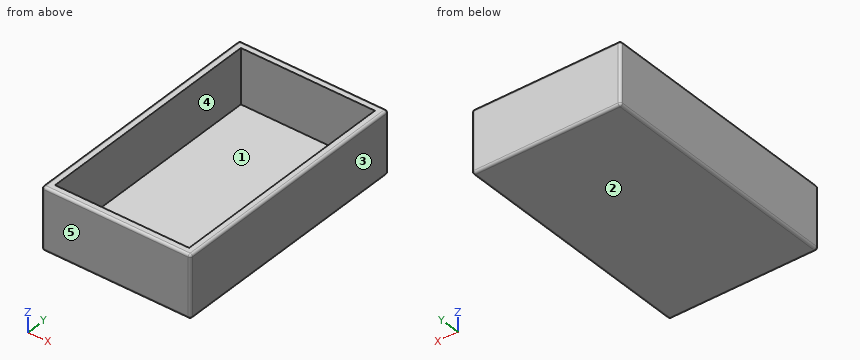
```python
from build123d import *

# Parameters (mm, degrees)
F0_W     = 60
F0_H     = 100
F1_DEPTH = 25
F2_T     = -3
F3_R     = 1


with BuildPart() as f1:
    # F0 (on Top) → F1 (new body)
    with BuildSketch(Plane.XY):
        with Locations((-16.971023, 0.550396)):
            Rectangle(F0_W, F0_H)
    extrude(amount=F1_DEPTH)

    # F2
    f2_openings = [f1.faces().sort_by_distance(p)[0] for p in [
        (-16.971023, 0.550396, 25),
    ]]
    offset(amount=F2_T, openings=f2_openings)

    # F3
    f3_edges = [f1.edges().sort_by_distance(p)[0] for p in [
        (13.028977, 0.550396, 25),
        (-16.971023, -49.449604, 25),
        (-46.971023, 0.550396, 25),
        (-16.971023, 50.550396, 25),
        (13.028977, 50.550396, 12.5),
        (13.028977, -49.449604, 12.5),
        (-46.971023, -49.449604, 12.5),
        (-16.971023, -49.449604, 0),
        (13.028977, 0.550396, 0),
        (-16.971023, 50.550396, 0),
        (-46.971023, 0.550396, 0),
        (-46.971023, 50.550396, 12.5),
    ]]
    fillet(f3_edges, radius=F3_R)


solid = f1.part
```
Could you check a few things on this model? Use its own coordinates, in mm. Face numbers are marked on the shaded views. A direction names the side the tool comes from. Round coordinates to 2 decimals unless told otherwise and drop trailing zeros. Loops run counter-clockwise (first coordinate to the right, second up) from the corner with the lowest first, then second, coordinate; pieces in that order, holes last. Notation, with made-up numbers: (43, 18.5) -> (98, 18.5) arc R10 ccw to (98, 33.5) -> close; hole circle Ø7 at (10, 1). An arc over 180 degrees is marked (long way). Put each result on its own line as item: value.
Q1. For pin 1 Ø12 at (x, y) = (-0.5, 10.5) entering from +Z, with a flat end and sliding along its axis, tell me the tip position at first contact or that it passes through.
Checks:
pin 1: z = 3
Q2. I want a section at A-A on z = 19. Write out the boundary of the cut face in (x, y).
Checks:
outline: (-46.97, -48.45) arc R1 ccw to (-45.97, -49.45) -> (12.03, -49.45) arc R1 ccw to (13.03, -48.45) -> (13.03, 49.55) arc R1 ccw to (12.03, 50.55) -> (-45.97, 50.55) arc R1 ccw to (-46.97, 49.55) -> close; hole (-43.97, -46.45) -> (10.03, -46.45) -> (10.03, 47.55) -> (-43.97, 47.55) -> close
Q3. Which directions (+Z, -Z, +X, -X, +Y, -Y) give clear straight access to the entire face, cutting with the end or side of a thin tool? Please do the marked faces 1 and 2.
Checks:
face 1: +Z
face 2: -Z, +X, -X, +Y, -Y
Q4. I want a section at C-C on x = -35.5. Write out the boundary of the cut face in (y, z).
Checks:
outline: (-49.45, 1) arc R1 ccw to (-48.45, 0) -> (49.55, 0) arc R1 ccw to (50.55, 1) -> (50.55, 24) arc R1 ccw to (49.55, 25) -> (47.55, 25) -> (47.55, 3) -> (-46.45, 3) -> (-46.45, 25) -> (-48.45, 25) arc R1 ccw to (-49.45, 24) -> close
Q5. I want a section at B-B on y = 39. Write out the boundary of the cut face in (x, z).
Checks:
outline: (-46.97, 1) arc R1 ccw to (-45.97, 0) -> (12.03, 0) arc R1 ccw to (13.03, 1) -> (13.03, 24) arc R1 ccw to (12.03, 25) -> (10.03, 25) -> (10.03, 3) -> (-43.97, 3) -> (-43.97, 25) -> (-45.97, 25) arc R1 ccw to (-46.97, 24) -> close
Q6. Please list where these lines run through material, in increasing order: line 1 (X direction, y = 2.5, z = 3.5); line 2 (Y direction, x = -1, z = 13.75); line 3 (Z direction, x = 0, y = 10.5). Write a range as from..to.
Checks:
line 1: -46.97..-43.97, 10.03..13.03
line 2: -49.45..-46.45, 47.55..50.55
line 3: 0..3
Q7. Thinking about a two-plate mould opening in X: for the marked faces 3, 4 and 5, which applies, pulls with the +X half, pulls with the -X half, needs draft (parallel to the pull), parting line crosses it, or undercut?
Checks:
face 3: pulls with the +X half
face 4: undercut
face 5: needs draft
